Here's how the part is built. I have some questions about the finished solid (model axes, mm). Give positions to 0.01 mm unless a question says otherwise; leave off trailing zeros. Loops run counter-clockwise (first coordinate to the right, second up) from the corner with the lowest first, then second, coordinate; pieces in that order, holes last. Notation, with made-up numbers: (47, 35) - (93, 35) arc R34 ccw to (93, 70) - close; hole circle Ø2 at (52, 89). An arc over 180 degrees is marked (long way). One line per item, written item: value. Start each with the question number.
```python
from build123d import *

# Parameters (mm, degrees)
F0_R     = 2.5
F1_DEPTH = 75
F2_R     = 2.5
F3_R     = 1.075
F4_DEPTH = 15
F5_R     = 0.5


with BuildPart() as f1:
    # F0 (on Top) → F1 (new body)
    with BuildSketch(Plane.XY):
        Circle(F0_R)
    extrude(amount=F1_DEPTH)

    # F2
    f2_edges = [f1.edges().sort_by_distance(p)[0] for p in [
        (-2.5, 0, 75),
    ]]
    fillet(f2_edges, radius=F2_R)

    # F3 (on face) → F4 (cut)
    with BuildSketch(Plane(origin=(0, 0, 0), x_dir=(1, 0, 0), z_dir=(0, 0, -1))):
        Circle(F3_R)
    extrude(amount=-F4_DEPTH, mode=Mode.SUBTRACT)

    # F5
    f5_edges = [f1.edges().sort_by_distance(p)[0] for p in [
        (-1.075, 0, 0),
        (1.075, 0, 7.5),
        (-1.075, 0, 15),
    ]]
    fillet(f5_edges, radius=F5_R)


solid = f1.part
```
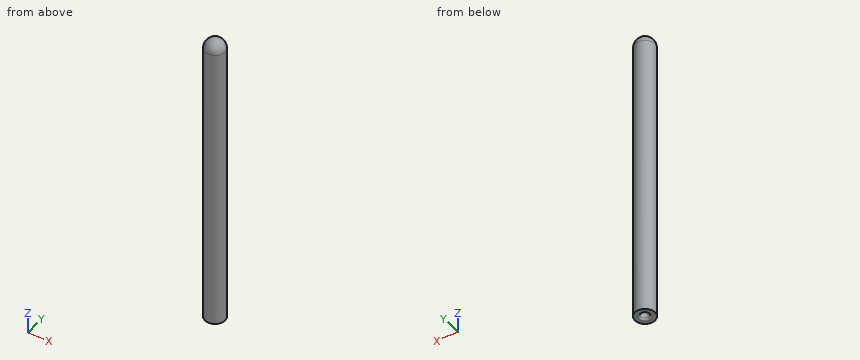
(1) Please list where these lines run through material, in increasing order: probe 1 along X at (y, z) = (-0.05, 7); probe 2 along Y at (x, z) = (0, 8.5) (3 decimals); probe 3 along Y at (x, z) = (2.25, 62). Write a range as from..to.
(2) Will these pins go through, and if not, where does the flat tip stop? pin 1 (1 mm diameter, centred on y = -2, z = 67.5, fed in from -X); pin 2 (2 mm diameter, centred on x = 1.5, z = 62, fed in from -Y); pin 3 (0.6 mm diameter, centred on x = 0, y = 0, fed in from -Z).
(3) If we section it at A-A on z = 12.5: List the corners of the cut face in (x, y) for me (3 decimals).
(4) If we section it at B-B on z = 30: List the corners of the cut face in (x, y) for me, plus the area to 3 significant figures.
Found:
1. probe 1: -2.5..-1.07, 1.07..2.5
1. probe 2: -2.5..-1.075, 1.075..2.5
1. probe 3: -1.09..1.09
2. pin 1: x = -2
2. pin 2: y = -2.45
2. pin 3: z = 15
3. outline: circle Ø5 at (0, 0); hole circle Ø2.15 at (0, 0)
4. outline: circle Ø5 at (0, 0)
4. area: 19.6 mm^2
